Answer from the drawing. Dimensions are ordinates in mm from the lowest x, y and z of the part. Coordinates: 2 decimals unless noted, no trailing zeros. Write each loop counter-clockwise with the first axis right and the second up, starting at its lowest first coordinate (ties: lowest second). Pieces come first, ordered by that corner, then holes. Notation, with made-up numbers: (44.5, 28.25) -> (58.5, 28.25) arc R8 ccw to (58.5, 32.25) -> close; hole circle Ø9 at (-20.5, 45). An arc over 180 degrees is marked (long way). Return JSON: item names as keys, results as strings.
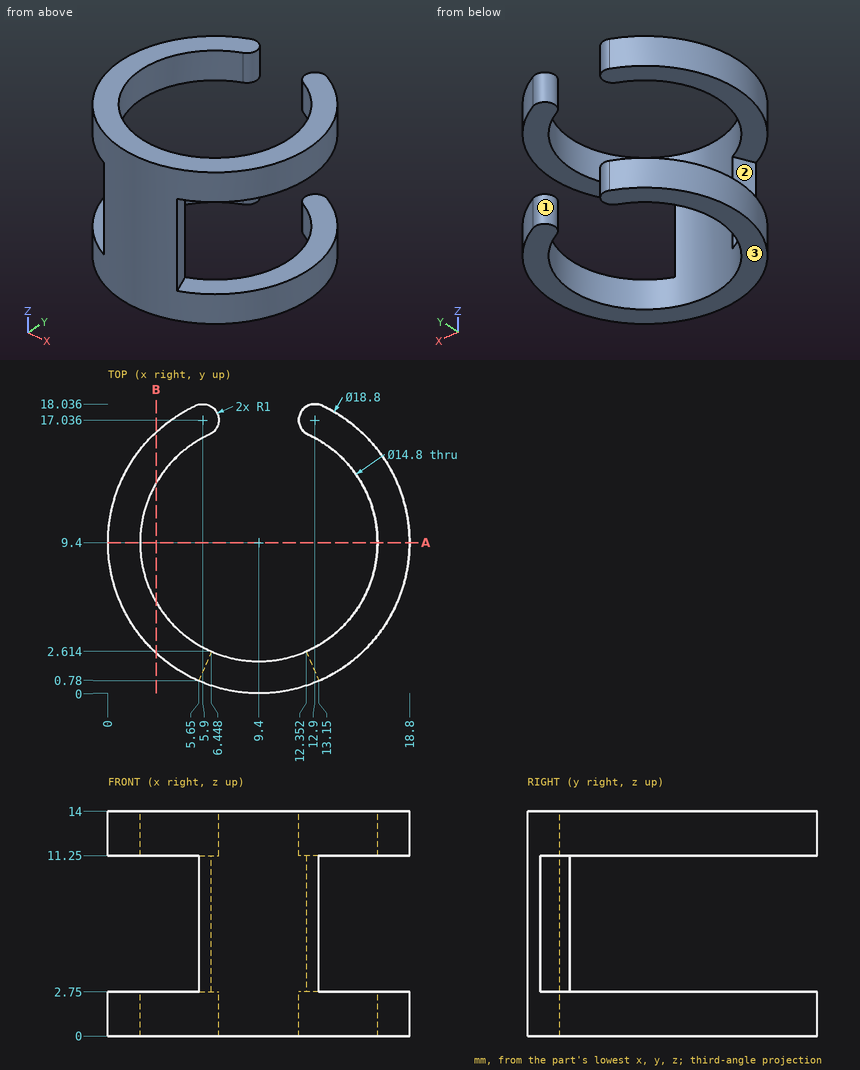
1. For a pull along X with two mould halves and no side action, classify the marked faces 1, 2 and 3 as +X half, -X half, draft (parallel to the pull), parting line (faces both ways), or undercut.
Taken from the geometry:
{"face 1": "undercut", "face 2": "-X half", "face 3": "draft"}
2. Flat-ended cylindrical pins translate along their axes: pin 1 Ø5 at (y, z) = (8, 10.5) entering from +X; pin 2 Ø4 at (x, z) = (7, 4.5) entering from -Y; pin 3 Ø3.5 at (x, y) = (5, 9) entering from -Z; pin 4 Ø3 at (x, z) = (11, 2.5) entering from +Y. Find the tip coordinate at first contact, or state that the pin passes through.
Taken from the geometry:
{"pin 1": "stops at x = 18.8", "pin 2": "stops at y = 0.01", "pin 3": "passes through", "pin 4": "stops at y = 17.95"}
3. The part is cut by section B-B (x = 3). Count the separate pieces of the cut face and the enclosed holes in it.
Taken from the geometry:
{"separate pieces": "4", "enclosed holes": "0"}
4. Consider L1, parallel to Z at x = 16.5, y = 7; L2, parallel to Y at x = 9.4, z = 8.5; L3, parallel to X at y = 8, z = 2.5 (1 decimal). Determine where each line is inside the solid, lowest interval first.
Taken from the geometry:
{"L1": "z = 0 to 2.75, 11.25 to 14", "L2": "y = 0 to 2", "L3": "x = 0.1 to 2.1, 16.7 to 18.7"}
5. The part is cut by section A-A (y = 9.4). Determine the outline of the cut face in (x, z).
Taken from the geometry:
{"outline": "(0, 0) -> (2, 0) -> (2, 2.75) -> (0, 2.75) -> close; (0, 11.25) -> (2, 11.25) -> (2, 14) -> (0, 14) -> close; (16.8, 0) -> (18.8, 0) -> (18.8, 2.75) -> (16.8, 2.75) -> close; (16.8, 11.25) -> (18.8, 11.25) -> (18.8, 14) -> (16.8, 14) -> close"}
